Autodesk Inventor part; units mm, degrees
ref_plane "Work Plane4" through (-50, 152.4, 0) normal (-1, 0, 0) x (0, -1, 0)
ref_plane "YZ Plane" through (0, 0, 0) normal (1, 0, 0) x (0, 1, 0)
ref_plane "XZ Plane" through (0, 0, 0) normal (0, 1, 0) x (-1, 0, 0)
sketch "Sketch1" plane through (0, 0, 0) normal (0, 1, 0) x (-1, 0, 0)
  circle A0 centre (0, 0) radius 50
  circle A1 centre (0, 0) radius 47.46
  dimension "d0" = 100
  dimension "d1" = 2.54
extrude "Extrusion1" add sketch "Sketch1" along normal blind 152.4
sketch "Sketch4" plane through (0, 152.4, 0) normal (0, 1, 0) x (1, 0, 0)
  circle A0 centre (0, 0) radius 47.46
  circle A1 centre (0, 0) radius 50
  point P0 (-50, 0)
ref_plane "Work Plane4" through (-50, 152.4, 0) normal (-1, 0, 0) x (0, -1, 0)
sketch "Sketch8" plane through (-50, 152.4, 0) normal (-1, 0, 0) x (0, -1, 0)
  line L0 (0, 0) -> (0, 304.8) construction
  arc A0 (-304.8, 304.8) -> (0, 0) centre (0, 304.8) ccw
  line L1 (0, 304.8) -> (-304.8, 304.8) construction
  point P0 (152.4, 0)
  dimension "d7" = 304.8
sweep "Sweep1" add profiles "Sketch4" path "Sketch8"
sketch "Sketch9" plane through (0, 457.2, 304.8) normal (0, 0, 1) x (1, 0, 0)
  circle A0 centre (0, 0) radius 47.46
  circle A1 centre (0, 0) radius 50
  point P0 (0, -457.2)
extrude "Extrusion2" add sketch "Sketch9" along normal blind 152.4
properties part number "sweep"
Work out the finished part from the listing and answer in its coordinate system (mm). A direction names the side the tool comes from. Round coordinates to 2 decimals unless told otherwise and drop trailing zeros. Order: outer loops, then holes, each group sorted by start corner. A loop starts at its lowest first (then second) coordinate and runs counter-clockwise, first axis right, second up.
Q1. The mould has two halves that part along Y. Classify faces 3 (the cylindrical face through (-10.84, 506.01, 379.93)), 4 (the cylindrical face through (-47.69, 75.13, -15.02)), 5 (the cylindrical face through (-10.29, 503.53, 379.93)): pulls with the +Y half, pulls with the -Y half, needs draft (parallel to the pull), parting line crosses it, or undercut.
Solution:
face 3: parting line crosses it
face 4: needs draft
face 5: undercut
Q2. A tool of negligible diameter and unlimited length cuts with its end or side. For faces 1 (the flat face through (-18.3, 0, -44.2)), 2 (the cylindrical face through (37.66, 75.13, 28.88)), from which of +Z, -Z, +X, -X, +Y, -Y can it reach the whole face along a straight path? Write none if from no direction.
Solution:
face 1: +Z, -Z, +X, -X, -Y
face 2: -Y
Q3. A cutting plane is placed at B-B, the plane x = -30.5. Determine the outline of the cut face in (y, z).
Solution:
outline: (0, -39.62) - (152.4, -39.62) arc R344.42 ccw to (496.82, 304.8) - (496.82, 457.2) - (493.56, 457.2) - (493.56, 304.8) arc R341.16 cw to (152.4, -36.36) - (0, -36.36) - close; (0, 36.36) - (152.4, 36.36) arc R268.44 ccw to (420.84, 304.8) - (420.84, 457.2) - (417.58, 457.2) - (417.58, 304.8) arc R265.18 cw to (152.4, 39.62) - (0, 39.62) - close
Q4. Given pin 1 Ø6 at (x, z) = (23.5, 336.5) entering from -Y; pin 2 Ø8 at (x, z) = (29, 150.5) entering from -Y; pin 3 Ø12 at (x, y) = (-22.5, 65.5) entering from +Z, each flat-ended and moving along its own axis, determine where each tip first touches the part or whether it passes through.
Solution:
pin 1: stops at y = 411.6
pin 2: stops at y = 362.3
pin 3: stops at z = 47.2
Q5. Find the intervals of material crossed by line 1 along X through (y, z) = (112, 0); line 2 along Y through (x, z) = (0, 356), in increasing order.
Solution:
line 1: x = -50 to -47.46, 47.46 to 50
line 2: y = 407.2 to 409.74, 504.66 to 507.2
Q6. A cutting plane is placed at A-A, the plane x = 0. Determine the outline of the cut face in (y, z).
Solution:
outline: (0, -50) - (152.4, -50) arc R354.8 ccw to (507.2, 304.8) - (507.2, 457.2) - (504.66, 457.2) - (504.66, 304.8) arc R352.26 cw to (152.4, -47.46) - (0, -47.46) - close; (0, 47.46) - (152.4, 47.46) arc R257.34 ccw to (409.74, 304.8) - (409.74, 457.2) - (407.2, 457.2) - (407.2, 304.8) arc R254.8 cw to (152.4, 50) - (0, 50) - close
